```python
from build123d import *

# Parameters (mm, degrees)
SKETCH2_R               = 2.5
BOSS_EXTRUDE1_DEPTH     = 52
SKETCH3_W               = 2.4
SKETCH3_H               = 5
CUT_EXTRUDE1_DEPTH      = 8
CUT_EXTRUDE2_DEPTH      = 53.120053722
CUT_EXTRUDE2_DEPTH_BACK = 53.120053722
SKETCH4_R               = 1.25
SKETCH5_W               = 2.4
SKETCH5_H               = 5
CUT_EXTRUDE3_DEPTH      = 8


with BuildPart() as part:
    # Sketch2 → Boss-Extrude1 (new body)
    with BuildSketch(Plane(origin=(0, 0, 0), x_dir=(-1, 0, 0), z_dir=(0, 1, 0))):
        with Locations(Location((0, 0, 0), (0, 0, 270))):
            Circle(SKETCH2_R)
    extrude(amount=BOSS_EXTRUDE1_DEPTH)

    # Sketch3 → Cut-Extrude1 (cut)
    with BuildSketch(Plane.XZ):
        Rectangle(SKETCH3_W, SKETCH3_H)
    extrude(amount=-CUT_EXTRUDE1_DEPTH, mode=Mode.SUBTRACT)

    # Sketch4 → Cut-Extrude2 (cut, two sides: drawn at the far end of the back side and taken through both)
    with BuildSketch(Plane.YZ.offset(-CUT_EXTRUDE2_DEPTH_BACK)):
        with Locations(Location((4, 0, 0), (0, 0, 270))):
            Circle(SKETCH4_R)
        with Locations(Location((48, 0, 0), (0, 0, 270))):
            Circle(SKETCH4_R)
    extrude(amount=CUT_EXTRUDE2_DEPTH + CUT_EXTRUDE2_DEPTH_BACK, mode=Mode.SUBTRACT)

    # Sketch5 → Cut-Extrude3 (cut)
    with BuildSketch(Plane(origin=(0, 52, 0), x_dir=(-1, 0, 0), z_dir=(0, 1, 0))):
        Rectangle(SKETCH5_W, SKETCH5_H)
    extrude(amount=-CUT_EXTRUDE3_DEPTH, mode=Mode.SUBTRACT)


solid = part.part
```
Work out the finished part from the listing and answer in its coordinate system (mm). A direction names the side the tool comes from. Round coordinates to 2 decimals unless told otherwise and drop trailing zeros. Order: outer loops, then holes, each group sorted by start corner. A loop starts at its lowest first (then second) coordinate and runs counter-clockwise, first axis right, second up.
Q1. Find the intervals of material crossed by line 1 along Y through (x, z) = (-2.1, 0); line 2 along X through (y, z) = (44.5, 1.2); line 3 along Y through (x, z) = (1.25, -0.6), in increasing order.
Solution:
line 1: y = 0 to 2.75, 5.25 to 46.75, 49.25 to 52
line 2: x = -2.19 to -1.2, 1.2 to 2.19
line 3: y = 0 to 2.9, 5.1 to 46.9, 49.1 to 52
Q2. A tool of negligible diameter and unlimited length cuts with its end or side. For faces 1 (the cylindrical face through (1.84, 47.24, 0.99)), 2 (the flat face through (-1.2, 47, -1)), 3 (the flat face through (-1.2, 5, -1)), from which of +Z, -Z, +X, -X, +Y, -Y can it reach the whole face along a straight path? Write none if from no direction.
Solution:
face 1: +X, -X
face 2: +Z, -Z, +Y
face 3: +Z, -Z, -Y
Q3. The mould has two halves that part along X. Classify faces 4 (the flat face through (0, 8, 0)), 5 (the cylindrical face through (-0.1, 25.6, 2.5)), 6 (the flat face through (1.2, 5, -1)), 7 (the flat face through (-2, 0, 0)): pulls with the +X half, pulls with the -X half, needs draft (parallel to the pull), parting line crosses it, or undercut.
Solution:
face 4: undercut
face 5: parting line crosses it
face 6: undercut
face 7: needs draft
Q4. A cutting plane is placed at B-B, the plane y = 46. Determine the outline of the cut face in (x, z).
Solution:
outline: (-1.2, -2.19) - (-1.2, 2.19) arc R2.5 ccw to start; (1.2, -2.19) arc R2.5 ccw to (1.2, 2.19) - close
Q5. Given pin 1 Ø3 at (y, z) = (48, 0) entering from -X; pin 2 Ø0.7 at (x, z) = (-0.5, 0.5) entering from -Y; pin 3 Ø0.7 at (x, z) = (-0.5, -0.5) entering from +Y, each flat-ended and moving along its own axis, determine where each tip first touches the part or whether it passes through.
Solution:
pin 1: stops at x = -2.5
pin 2: stops at y = 8
pin 3: stops at y = 44
Q6. A cutting plane is placed at A-A, the plane z = 0. Determine the outline of the cut face in (x, y).
Solution:
outline: (-2.5, 0) - (-1.2, 0) - (-1.2, 2.75) - (-2.5, 2.75) - close; (-2.5, 5.25) - (-1.2, 5.25) - (-1.2, 8) - (1.2, 8) - (1.2, 5.25) - (2.5, 5.25) - (2.5, 46.75) - (1.2, 46.75) - (1.2, 44) - (-1.2, 44) - (-1.2, 46.75) - (-2.5, 46.75) - close; (-2.5, 49.25) - (-1.2, 49.25) - (-1.2, 52) - (-2.5, 52) - close; (1.2, 0) - (2.5, 0) - (2.5, 2.75) - (1.2, 2.75) - close; (1.2, 49.25) - (2.5, 49.25) - (2.5, 52) - (1.2, 52) - close
Q7. A cutting plane is placed at C-C, the plane y = 37. Determine the outline of the cut face in (x, z).
Solution:
outline: circle Ø5 at (0, 0)
Q8. A cutting plane is placed at D-D, the plane x = -0.5. Determine the outline of the cut face in (y, z), then the cut area to 3 significant figures.
Solution:
outline: (8, -2.45) - (44, -2.45) - (44, 2.45) - (8, 2.45) - close
area: 176 mm2
